Geometry check sheet. Reference: drawing and pictorial views, mm from the part's lowest x, y, z. Give positions to 0.01 mm unless a question says otherwise; leave off trailing zeros. Write each loop counter-clockwise with the first axis right and the second up, starting at its lowest first coordinate (ties: lowest second). Pieces come first, ordered by that corner, then holes. Notation, with made-up numbers: (37, 24.5) -> (84, 24.5) arc R34 ccw to (84, 55.5) -> close; hole circle Ø2 at (56, -15.75). An arc over 180 degrees is marked (long way). Return JSON: item names as keys, results as strings.
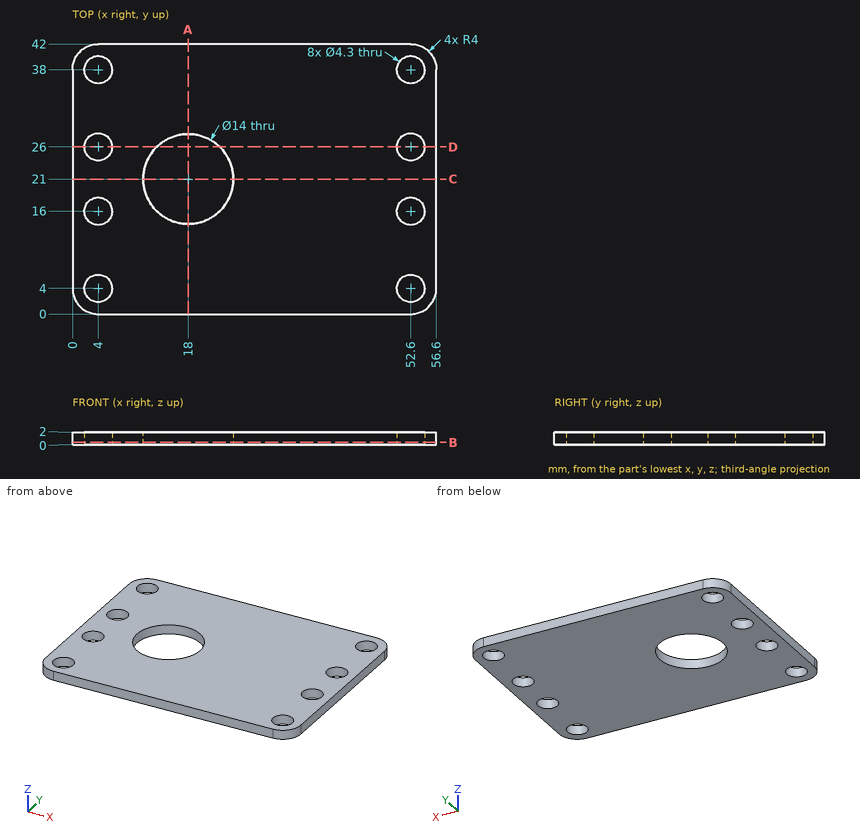
(1) Cross-section at B-B on z = 0.4. State how many separate pieces and enclosed holes the cut face has, then the cut area to 3 significant figures.
Reply:
{"separate pieces": "1", "enclosed holes": "9", "area": "2,090 mm^2"}
(2) Thickness scan on L1, parallel to Y at x = 4, z = 0.6; L2, parallel to X at y = 38, z = 0.45; L3, parallel to X at y = 36.5, z = 1.55. Record the ranges inside material, lowest first.
Reply:
{"L1": "0 to 1.85, 6.15 to 13.85, 18.15 to 23.85, 28.15 to 35.85, 40.15 to 42", "L2": "0 to 1.85, 6.15 to 50.45, 54.75 to 56.6", "L3": "0 to 2.46, 5.54 to 51.06, 54.14 to 56.6"}
(3) Depth check by flat-ended pin: pin 1 Ø2.5 at (x, y) = (52.6, 26) entering from +Z. Enter the tip coordinate at first touch or a pass-through.
Reply:
{"pin 1": "through"}
(4) Cross-section at A-A on x = 18. Enter the section's corners in (y, z).
Reply:
{"outline": "(0, 0) -> (14, 0) -> (14, 2) -> (0, 2) -> close; (28, 0) -> (42, 0) -> (42, 2) -> (28, 2) -> close"}
(5) Cross-section at C-C on y = 21. Enter the section's corners in (x, z), then the cut area to 3 significant figures.
Reply:
{"outline": "(0, 0) -> (11, 0) -> (11, 2) -> (0, 2) -> close; (25, 0) -> (56.6, 0) -> (56.6, 2) -> (25, 2) -> close", "area": "85.2 mm^2"}
(6) Cross-section at D-D on y = 26. Enter the section's corners in (x, z).
Reply:
{"outline": "(0, 0) -> (1.85, 0) -> (1.85, 2) -> (0, 2) -> close; (6.15, 0) -> (13.1, 0) -> (13.1, 2) -> (6.15, 2) -> close; (22.9, 0) -> (50.45, 0) -> (50.45, 2) -> (22.9, 2) -> close; (54.75, 0) -> (56.6, 0) -> (56.6, 2) -> (54.75, 2) -> close"}
